from build123d import *

# Parameters (mm, degrees)
SKETCH1_R               = 55
BOSS_EXTRUDE1_DEPTH     = 200
SKETCH2_R               = 51
CUT_EXTRUDE1_DEPTH      = 190
SKETCH3_R               = 19
CUT_EXTRUDE2_DEPTH      = 1
CUT_EXTRUDE2_DEPTH_BACK = 201
SKETCH4_R               = 5
CUT_EXTRUDE3_DEPTH      = 2
SKETCH5_R               = 22.5
CUT_EXTRUDE4_DEPTH      = 2
CUT_SWEEP1_PROFILE_R    = 2.5
SKETCH58_R              = 2.5
CUT_EXTRUDE5_DEPTH      = 2


with BuildPart() as part:
    # Sketch1 → Boss-Extrude1 (new body)
    with BuildSketch(Plane(origin=(0, 0, 0), x_dir=(0, 0, -1), z_dir=(1, 0, 0))):
        Circle(SKETCH1_R)
    extrude(amount=BOSS_EXTRUDE1_DEPTH)

    # Sketch2 → Cut-Extrude1 (cut)
    with BuildSketch(Plane(origin=(200, 0, 0), x_dir=(0, 0, -1), z_dir=(1, 0, 0))):
        Circle(SKETCH2_R)
    extrude(amount=-CUT_EXTRUDE1_DEPTH, mode=Mode.SUBTRACT)

    # Sketch3 → Cut-Extrude2 (cut, two sides)
    with BuildSketch(Plane.ZY) as cut_extrude2_sk:
        Circle(SKETCH3_R)
    extrude(amount=CUT_EXTRUDE2_DEPTH, mode=Mode.SUBTRACT)
    extrude(cut_extrude2_sk.sketch, amount=-CUT_EXTRUDE2_DEPTH_BACK, mode=Mode.SUBTRACT)

    # Sketch4 → Cut-Extrude3 (cut)
    with BuildSketch(Plane.ZY):
        with Locations((0, 34)):
            Circle(SKETCH4_R)
        with Locations((0, -34)):
            Circle(SKETCH4_R)
    extrude(amount=-CUT_EXTRUDE3_DEPTH, mode=Mode.SUBTRACT)

    # Sketch5 → Cut-Extrude4 (cut)
    with BuildSketch(Plane.ZY):
        Circle(SKETCH5_R)
    extrude(amount=-CUT_EXTRUDE4_DEPTH, mode=Mode.SUBTRACT)

    # Cut-Sweep1: sweep along a path in Sketch57
    with BuildLine(Plane(origin=(105, 0, 0), x_dir=(0, 0, -1), z_dir=(1, 0, 0))) as cut_sweep1_path:
        CenterArc((0, 0), 55, 0, 360)
    # Cut-Sweep1 profile (on start of the path) → Cut-Sweep1 (sweep, cut)
    with BuildSketch(Plane(origin=(105, 0, -55), x_dir=(0, 0, 1), z_dir=(0, 1, 0))):
        Circle(CUT_SWEEP1_PROFILE_R)
    sweep(path=cut_sweep1_path.line, mode=Mode.SUBTRACT)

    # Sketch58 → Cut-Extrude5 (cut)
    with BuildSketch(Plane.ZY.offset(-2)):
        with Locations((0, 34)):
            Circle(SKETCH58_R)
        with Locations((0, -34)):
            Circle(SKETCH58_R)
    extrude(amount=-CUT_EXTRUDE5_DEPTH, mode=Mode.SUBTRACT)


solid = part.part
The model under review builds one solid part; all positions refer to its coordinate system, in mm. A direction names the side the tool comes from. Round coordinates to 2 decimals unless told otherwise and drop trailing zeros. Order: outer loops, then holes, each group sorted by start corner. A loop starts at its lowest first (then second) coordinate and runs counter-clockwise, first axis right, second up. Notation, with made-up numbers: (-15, 53) -> (23, 53) arc R18 cw to (23, 70) -> close; hole circle Ø3 at (55.25, 19.5). An arc over 180 degrees is marked (long way). Write item = value, one per line. Start each with the question number.
Item 1: Mouldability with a two-part tool opening along Y and no side actions: class faces 1 (the face through (2, 32, 2)), 2 (the face through (153.102, -53.692, 11.923)), 3 (the face through (0, -24, 1)) as released by +Y, released by -Y, zero draft, split by the parting line, or undercut.
Item 2: Consider section B-B on x = 180. Write out the cut boundary in (y, z).
Item 3: For faces 4 (the face through (106.33, -49.787, 11.056)), 5 (the face through (2.99, 36.11, 1.34)), 6 (the face through (5.944, -16.856, 8.767)), list the 3-axis set-ups (+Z, -Z, +X, -X, +Y, -Y) from which the entire face can be reached by the end or side of a thin tool; tool diameter is ignored.
Item 4: For line 1 along Y through (x, z) = (1.3, 0); line 2 along Y through (x, z) = (3, 0); line 3 along Y through (x, z) = (63.5, 0), list the stretches that pass through material, from the lowest coordinate up.
Item 5: Consider section A-A on y = 0. Write out the cut boundary in (x, z), plus the area to 3 significant figures.
Item 6: Clearance check with flat-ended pins moving along their axes: pin 1 Ø1 at (y, z) = (-39.5, 6.5) entering from -X; pin 2 Ø8 at (x, z) = (122, -41) entering from +Y; pin 3 Ø8 at (y, z) = (34, 0) entering from -X; pin 4 Ø5 at (x, y) = (155.5, 23.5) entering from -Z. State where each tip first meets the part, or that it passes through.
Conclusion:
q1.face_1 = undercut
q1.face_2 = split by the parting line
q1.face_3 = zero draft
q2.outline = circle Ø110 at (0, 0); hole circle Ø102 at (0, 0)
q3.face_4 = +X
q3.face_5 = -X
q3.face_6 = +X, -X
q4.line_1 = -55 to -39, -29 to -22.5, 22.5 to 29, 39 to 55
q4.line_2 = -55 to -36.5, -31.5 to -19, 19 to 31.5, 36.5 to 55
q4.line_3 = -55 to -51, 51 to 55
q5.outline = (0, -55) -> (102.5, -55) arc R2.5 cw to (107.5, -55) -> (200, -55) -> (200, -51) -> (10, -51) -> (10, -19) -> (2, -19) -> (2, -22.5) -> (0, -22.5) -> close; (0, 22.5) -> (2, 22.5) -> (2, 19) -> (10, 19) -> (10, 51) -> (200, 51) -> (200, 55) -> (107.5, 55) arc R2.5 cw to (102.5, 55) -> (0, 55) -> close
q5.area = 2,210 mm2
q6.pin_1 = 0
q6.pin_2 = 40.69
q6.pin_3 = 2
q6.pin_4 = -50.83
